Part model, mm, in its own coordinate system. Round coordinates to 2 decimals unless told otherwise and drop trailing zeros. Loops run counter-clockwise (first coordinate to the right, second up) from the corner with the lowest first, then second, coordinate; pieces in that order, holes last. Notation, with made-up numbers: M -1,36 L 46,36 A12 cw 46,41 Z; hole C 53,-24.5 d8. An arc over 180 degrees is marked long. Put each result on its own line as item: value. Start each with the question number.
```python
from build123d import *

# Parameters (mm, degrees)
SKETCH_1_R                           = 75
EXTRUDE_1_DEPTH                      = 3
SKETCH_2_R                           = 1.65
CUT_EXTRUDE_1_DEPTH                  = 107.108435103
CHAMFER_1_SIZE                       = 1.7
PATTERN_CIRCULAR_1_COUNT             = 3
CHAMFER_1_OF_PATTERN_CIRCULAR_1_SIZE = 1.7
SKETCH_3_R                           = 6.35
CUT_EXTRUDE_2_DEPTH                  = 107.108435103
CHAMFER_2_SIZE                       = 1


with BuildPart() as part:
    # Эскиз1 → Бобышка-Вытянуть1 (new body)
    with BuildSketch(Plane(origin=(0, 0, 0), x_dir=(1, 0, 0), z_dir=(0, 1, 0))):
        with Locations(Location((0, 0, 0), (0, 0, 270))):
            Circle(SKETCH_1_R)
    extrude(amount=EXTRUDE_1_DEPTH)

    # Эскиз2 → Вырез-Вытянуть1 (cut, through all)
    with BuildSketch(Plane(origin=(0, 3, 0), x_dir=(1, 0, 0), z_dir=(0, 1, 0))):
        with Locations(Location((0, 69.55, 0), (0, 0, 270))):
            Circle(SKETCH_2_R)
    cut_extrude_1 = extrude(amount=-CUT_EXTRUDE_1_DEPTH, mode=Mode.SUBTRACT)

    # Фаска1
    chamfer_1_edges = [part.edges().sort_by_distance(p)[0] for p in [
        (0, 3, -71.2),
    ]]
    chamfer(chamfer_1_edges, length=CHAMFER_1_SIZE)

    # Круговой массив1: Вырез-Вытянуть1 ×3 about axis
    pattern_circular_1_axis = Axis((0, 0, 0), (0, 1, 0))
    for i in range(1, PATTERN_CIRCULAR_1_COUNT):
        add(cut_extrude_1.rotate(pattern_circular_1_axis, i * 360 / PATTERN_CIRCULAR_1_COUNT), mode=Mode.SUBTRACT)

    # Фаска1 of Круговой массив1
    chamfer_1_of_pattern_circular_1_edges = [part.edges().sort_by_distance(p)[0] for p in [
        (-61.661008749, 3, 35.6),
        (61.661008749, 3, 35.6),
    ]]
    chamfer(chamfer_1_of_pattern_circular_1_edges, length=CHAMFER_1_OF_PATTERN_CIRCULAR_1_SIZE)

    # Эскиз3 → Вырез-Вытянуть2 (cut, through all)
    with BuildSketch(Plane(origin=(0, 3, 0), x_dir=(1, 0, 0), z_dir=(0, 1, 0))):
        with Locations(Location((0, 0, 0), (0, 0, 270))):
            Circle(SKETCH_3_R)
    extrude(amount=-CUT_EXTRUDE_2_DEPTH, mode=Mode.SUBTRACT)

    # Фаска2
    chamfer_2_edges = [part.edges().sort_by_distance(p)[0] for p in [
        (0, 3, -75),
    ]]
    chamfer(chamfer_2_edges, length=CHAMFER_2_SIZE)


solid = part.part
```
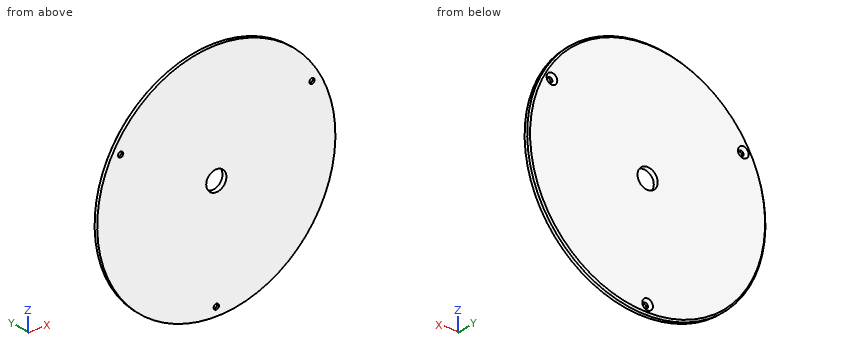
1. Drop flat-ended pins along their axis: pin 1 (1 mm diameter, centred on y = 1, z = -44, fed in from +X); pin 2 (2 mm diameter, centred on x = 60.23, z = 34.78, fed in from -Y); pin 3 (4.5 mm diameter, centred on x = -60.23, z = 34.77, fed in from +Y). Give the stop position or say it passes through.
2. Cut at A-A, the plane z = 0. Give the cut face in (x, y), and give its area (3 significant figures).
3. Wall check: L1, parallel to X at y = 1, z = 0; L2, parallel to Z at x = -45.5, y = 2.85; L3, parallel to X at y = 2.1, z = 0. Give the ranges that are in metal, low to high.
Results list:
1. pin 1: stops at x = 61.1
1. pin 2: passes through
1. pin 3: stops at y = 1.91
2. outline: M -75,0 L -6.35,0 L -6.35,3 L -74,3 L -75,2 Z; M 6.35,0 L 75,0 L 75,2 L 74,3 L 6.35,3 Z
2. area: 411 mm^2
3. L1: x = -75 to -6.35, 6.35 to 75
3. L2: z = -58.55 to 58.55
3. L3: x = -74.9 to -6.35, 6.35 to 74.9
